Model file for the job. Use its own axes, mm. Face numbers are marked on the shaded views. Round coordinates to 2 decimals unless told otherwise and drop trailing zeros. Loops run counter-clockwise (first coordinate to the right, second up) from the corner with the lowest first, then second, coordinate; pieces in that order, holes last. Notation, with made-up numbers: M 44.5,82.25 L 98.5,82.25 A12 cw 98.5,104.25 Z; hole C 2,43.5 d11. An arc over 180 degrees is marked long. Use a Markdown table: item, result. Add a question column.
Q1. Cut at C-C (x = 4.5). Give the cut face in (y, z), plus the area to 3 significant figures.
Q2. Cut at D-D (z = -3.05). Give the cut face in (x, y), plus the area to 3 significant figures.
Q3. Mould opens along Z. For the marked faces 1, 2 and 3 say: +Z half, -Z half, draft (parallel to the pull), parting line (faces both ways), or undercut.
Q4. Probe line 1 (Y direction, x = 0, z = -1.75); line 2 (Z direction, x = -4, y = -1.75); line 3 (Y direction, x = 0, z = -3.95). List the from-to ranges inside material, lowest first. Write a range as from..to.
Q5. Pin check, flat tips, straight feed: pin 1 (1.5 mm diameter, centred on y = -4, z = -2.5, fed in from -X); pin 2 (5 mm diameter, centred on x = 0, y = 2, fed in from +Z); pin 3 (1 mm diameter, centred on x = 3.5, z = -3, fed in from -Y). Stop position of each tip, or through.
Q6. Cut at A-A (y = 0). Give the cut face in (x, z), plus the area to 3 significant figures.
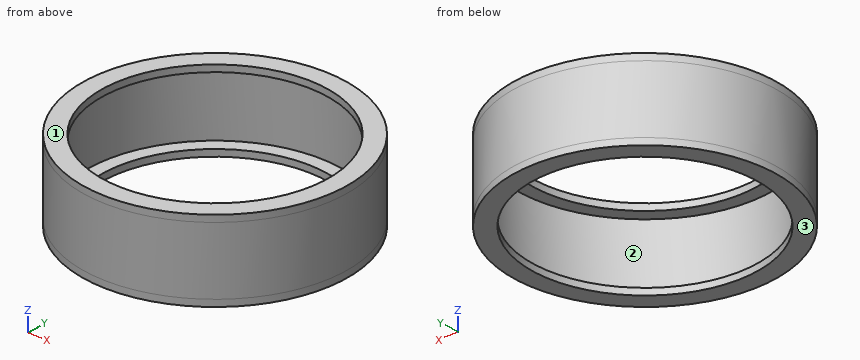
from build123d import *

# Parameters (mm, degrees)
SKETCH2_R           = 8.6106
BOSS_EXTRUDE1_DEPTH = 4.064
SKETCH3_R           = 10.033
BOSS_EXTRUDE2_DEPTH = 5.08
SKETCH4_R           = 8.6106
CUT_EXTRUDE1_DEPTH  = 6.08
SKETCH9_R           = 10.033
SKETCH9_R_2         = 8.128
BOSS_EXTRUDE3_DEPTH = 0.508
SKETCH10_R          = 10.033
SKETCH10_R_2        = 8.128
BOSS_EXTRUDE4_DEPTH = 0.508
SKETCH12_R          = 9.271
CUT_EXTRUDE2_DEPTH  = 7.096
SKETCH13_R          = 10.033
CUT_EXTRUDE3_DEPTH  = 0.508
SKETCH15_R          = 10.033
SKETCH15_R_2        = 9.271
CUT_EXTRUDE4_DEPTH  = 0.508
SKETCH16_R          = 9.652
SKETCH16_R_2        = 9.271
CUT_EXTRUDE5_DEPTH  = 6.08
SKETCH17_R          = 10.033
SKETCH17_R_2        = 8.6106
BOSS_EXTRUDE5_DEPTH = 0.508
SKETCH18_R          = 10.033
SKETCH18_R_2        = 8.6106
BOSS_EXTRUDE6_DEPTH = 0.508
SCALE1_SCALE        = 0.5


with BuildPart() as part:
    # Sketch2 → Boss-Extrude1 (new body)
    with BuildSketch(Plane.XY):
        Circle(SKETCH2_R)
    extrude(amount=-BOSS_EXTRUDE1_DEPTH)

    # Sketch3 → Boss-Extrude2 (add)
    with BuildSketch(Plane.XY):
        Circle(SKETCH3_R)
    extrude(amount=-BOSS_EXTRUDE2_DEPTH)

    # Sketch4 → Cut-Extrude1 (cut, through all)
    with BuildSketch(Plane.XY):
        Circle(SKETCH4_R)
    extrude(amount=-CUT_EXTRUDE1_DEPTH, mode=Mode.SUBTRACT)

    # Sketch9 → Boss-Extrude3 (add)
    with BuildSketch(Plane.XY):
        Circle(SKETCH9_R)
        Circle(SKETCH9_R_2, mode=Mode.SUBTRACT)
    extrude(amount=BOSS_EXTRUDE3_DEPTH)

    # Sketch10 → Boss-Extrude4 (add)
    with BuildSketch(Plane(origin=(0, 0, -5.08), x_dir=(-1, 0, 0), z_dir=(0, 0, -1))):
        Circle(SKETCH10_R)
        Circle(SKETCH10_R_2, mode=Mode.SUBTRACT)
    extrude(amount=BOSS_EXTRUDE4_DEPTH)

    # Sketch12 → Cut-Extrude2 (cut, through all)
    with BuildSketch(Plane(origin=(0, 0, -5.588), x_dir=(-1, 0, 0), z_dir=(0, 0, -1))):
        Circle(SKETCH12_R)
    extrude(amount=-CUT_EXTRUDE2_DEPTH, mode=Mode.SUBTRACT)

    # Sketch13 → Cut-Extrude3 (cut)
    with BuildSketch(Plane(origin=(0, 0, -5.588), x_dir=(-1, 0, 0), z_dir=(0, 0, -1))):
        Circle(SKETCH13_R)
    extrude(amount=-CUT_EXTRUDE3_DEPTH, mode=Mode.SUBTRACT)

    # Sketch15 → Cut-Extrude4 (cut)
    with BuildSketch(Plane.XY.offset(0.508)):
        Circle(SKETCH15_R)
        Circle(SKETCH15_R_2, mode=Mode.SUBTRACT)
    extrude(amount=-CUT_EXTRUDE4_DEPTH, mode=Mode.SUBTRACT)

    # Sketch16 → Cut-Extrude5 (cut, through all)
    with BuildSketch(Plane.XY):
        Circle(SKETCH16_R)
        Circle(SKETCH16_R_2, mode=Mode.SUBTRACT)
    extrude(amount=-CUT_EXTRUDE5_DEPTH, mode=Mode.SUBTRACT)

    # Sketch17 → Boss-Extrude5 (add)
    with BuildSketch(Plane.XY):
        Circle(SKETCH17_R)
        Circle(SKETCH17_R_2, mode=Mode.SUBTRACT)
    extrude(amount=BOSS_EXTRUDE5_DEPTH)

    # Sketch18 → Boss-Extrude6 (add)
    with BuildSketch(Plane(origin=(0, 0, -5.08), x_dir=(-1, 0, 0), z_dir=(0, 0, -1))):
        Circle(SKETCH18_R)
        Circle(SKETCH18_R_2, mode=Mode.SUBTRACT)
    extrude(amount=BOSS_EXTRUDE6_DEPTH)


with BuildPart() as part_1:
    # Scale1: scaled about (0, 0, -2.54)
    add(part.part.scale(SCALE1_SCALE).moved(Location((0, 0, -1.27))))


solid = part_1.part
Checked values:
| question | item | result |
|---|---|---|
| 1 | outline | M -2.22,-4.06 L 2.22,-4.06 L 2.22,-1.02 L -2.22,-1.02 Z; hole M -1.74,-3.81 L 1.74,-3.81 L 1.74,-1.27 L -1.74,-1.27 Z |
| 1 | area | 4.66 mm^2 |
| 2 | outline | C 0,0 d10.03; hole C 0,0 d9.65 |
| 2 | area | 5.89 mm^2 |
| 3 | face 1 | +Z half |
| 3 | face 2 | undercut |
| 3 | face 3 | -Z half |
| 4 | line 1 | y = -5.02..-4.83, 4.83..5.02 |
| 4 | line 2 | z = -4.06..-3.81, -1.27..-1.02 |
| 4 | line 3 | y = -5.02..-4.31, 4.31..5.02 |
| 5 | pin 1 | stops at x = -3.82 |
| 5 | pin 2 | stops at z = -1.02 |
| 5 | pin 3 | stops at y = -4.02 |
| 6 | outline | M -5.02,-4.06 L -4.31,-4.06 L -4.31,-3.81 L -4.83,-3.81 L -4.83,-1.27 L -4.31,-1.27 L -4.31,-1.02 L -5.02,-1.02 Z; M 4.31,-4.06 L 5.02,-4.06 L 5.02,-1.02 L 4.31,-1.02 L 4.31,-1.27 L 4.83,-1.27 L 4.83,-3.81 L 4.31,-3.81 Z |
| 6 | area | 1.69 mm^2 |
